Verification items for the finished model (mm, model axes). Coordinates: 2 decimals unless noted, no trailing zeros. Write each loop counter-clockwise with the first axis right and the second up, starting at its lowest first coordinate (ties: lowest second). Pieces come first, ordered by that corner, then holes. Notation, with made-up numbers: (-14.75, 57) -> (2.25, 57) arc R15 cw to (2.25, 71) -> close; hole circle Ø5 at (24.5, 5.5). An arc over 180 degrees is marked (long way). Write item = value, one per line. Start each with the question number.
(1) Section check A-A (y = 108). Record the cut outline in (x, z), plus the area to 3 significant figures.
(2) Material ranges on probe 1 along X at (y, z) = (466, 1.35); probe 2 along Y at (x, z) = (5, 3.15); probe 3 along X at (y, z) = (321, 2.1), recorded low to high. Write a range as [from, to].
(3) Gauge pin test, flat end, axial feed: pin 1 Ø2.5 at (x, y) = (160, 208) entering from -Z. Record the tip position at first contact, or that the pin passes through.
(4) Section check B-B (y = 443). Record the cut outline in (x, z).
(5) Section check C-C (z = 2.2). State how many separate pieces and enclosed holes the cut face has, plus the area to 3 significant figures.
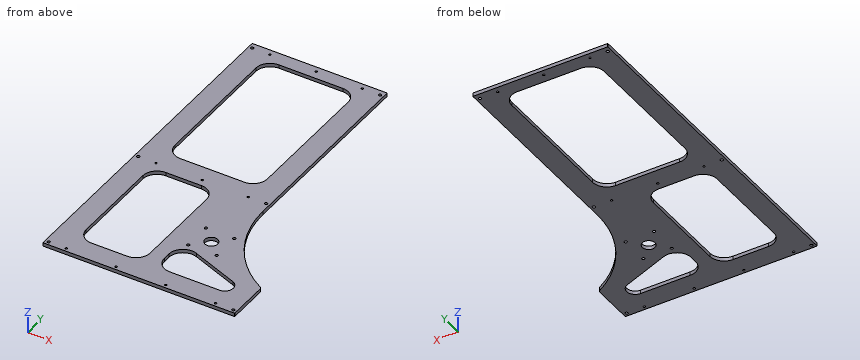
```python
from build123d import *

# Parameters (mm, degrees)
SKETCH1_R          = 9
EXTRUDE1_DEPTH     = 5
SKETCH2_R          = 2
SKETCH2_R_2        = 1.5
CUT_EXTRUDE1_DEPTH = 546.528184423
FILLET1_R          = 3
FILLET2_R          = 0.5
SKETCH3_R          = 2
CUT_EXTRUDE2_DEPTH = 546.528184423


with BuildPart() as part:
    # Sketch1 → Extrude1 (new body)
    with BuildSketch(Plane.XY):
        with BuildLine():
            Line((0, 0), (0, 474))
            Line((0, 474), (190, 474))
            Line((190, 474), (190, 193))
            ThreePointArc((190, 193), (211.541001234, 115.396842848), (270, 60))
            Line((270, 60), (270, 0))
            Line((270, 0), (0, 0))
        make_face()
        with Locations((170, 108)):
            Circle(SKETCH1_R, mode=Mode.SUBTRACT)
        with BuildLine():
            Line((30, 434), (30, 251))
            ThreePointArc((30, 251), (35.857864376, 236.857864376), (50, 231))
            Line((50, 231), (140, 231))
            ThreePointArc((140, 231), (154.142135624, 236.857864376), (160, 251))
            Line((160, 251), (160, 434))
            ThreePointArc((160, 434), (154.142135624, 448.142135624), (140, 454))
            Line((140, 454), (50, 454))
            ThreePointArc((50, 454), (35.857864376, 448.142135624), (30, 434))
        make_face(mode=Mode.SUBTRACT)
        with BuildLine():
            Line((30, 178), (30, 50))
            ThreePointArc((30, 50), (35.857864376, 35.857864376), (50, 30))
            Line((50, 30), (100, 30))
            ThreePointArc((100, 30), (114.142135624, 35.857864376), (120, 50))
            Line((120, 50), (120, 178))
            ThreePointArc((120, 178), (114.142135624, 192.142135624), (100, 198))
            Line((100, 198), (50, 198))
            ThreePointArc((50, 198), (35.857864376, 192.142135624), (30, 178))
        make_face(mode=Mode.SUBTRACT)
        with BuildLine():
            Line((160, 30), (230, 30))
            ThreePointArc((230, 30), (241.803319166, 39.836286369), (234.256500428, 53.219723887))
            Line((234.256500428, 53.219723887), (167.09416738, 78.699539812))
            ThreePointArc((167.09416738, 78.699539812), (148.639615931, 76.460306006), (140, 60))
            Line((140, 60), (140, 50))
            ThreePointArc((140, 50), (145.857864376, 35.857864376), (160, 30))
        make_face(mode=Mode.SUBTRACT)
    extrude(amount=EXTRUDE1_DEPTH)

    # Sketch2 → Cut-Extrude1 (cut, through all)
    with BuildSketch(Plane.XY.offset(5)):
        with Locations((185, 466)):
            Circle(SKETCH2_R)
        with Locations((5, 466)):
            Circle(SKETCH2_R)
        with Locations((5, 208)):
            Circle(SKETCH2_R)
        with Locations((5, 5)):
            Circle(SKETCH2_R)
        with Locations((265, 5)):
            Circle(SKETCH2_R)
        with Locations((185, 208)):
            Circle(SKETCH2_R)
        with Locations((30, 5)):
            Circle(SKETCH2_R_2)
        with Locations((100, 5)):
            Circle(SKETCH2_R_2)
        with Locations((170, 5)):
            Circle(SKETCH2_R_2)
        with Locations((240, 5)):
            Circle(SKETCH2_R_2)
        with Locations((30, 208)):
            Circle(SKETCH2_R_2)
        with Locations((95, 208)):
            Circle(SKETCH2_R_2)
        with Locations((160, 208)):
            Circle(SKETCH2_R_2)
        with Locations((30, 466)):
            Circle(SKETCH2_R_2)
        with Locations((95, 466)):
            Circle(SKETCH2_R_2)
        with Locations((160, 466)):
            Circle(SKETCH2_R_2)
    extrude(amount=-CUT_EXTRUDE1_DEPTH, mode=Mode.SUBTRACT)

    # Fillet1
    fillet1_edges = [part.edges().sort_by_distance(p)[0] for p in [
        (270, 60, 2.5),
    ]]
    fillet(fillet1_edges, radius=FILLET1_R)

    # Fillet2
    fillet2_edges = [part.edges().sort_by_distance(p)[0] for p in [
        (190, 474, 2.5),
        (270, 0, 2.5),
        (0, 0, 2.5),
        (0, 474, 2.5),
    ]]
    fillet(fillet2_edges, radius=FILLET2_R)

    # Sketch3 → Cut-Extrude2 (cut, through all)
    with BuildSketch(Plane.XY.offset(5)):
        with Locations((150, 128)):
            Circle(SKETCH3_R)
        with Locations((190, 128)):
            Circle(SKETCH3_R)
        with Locations((150, 88)):
            Circle(SKETCH3_R)
        with Locations((190, 88)):
            Circle(SKETCH3_R)
    extrude(amount=-CUT_EXTRUDE2_DEPTH, mode=Mode.SUBTRACT)


solid = part.part
```
Response:
q1.outline = (0, 0) -> (30, 0) -> (30, 5) -> (0, 5) -> close; (120, 0) -> (161, 0) -> (161, 5) -> (120, 5) -> close; (179, 0) -> (216.29, 0) -> (216.29, 5) -> (179, 5) -> close
q1.area = 541 mm2
q2.probe_1 = [0, 3], [7, 28.5], [31.5, 93.5], [96.5, 158.5], [161.5, 183], [187, 190]
q2.probe_2 = [0, 3], [7, 206], [210, 464], [468, 474]
q2.probe_3 = [0, 30], [160, 190]
q3.pin_1 = through
q4.outline = (0, 0) -> (32.14, 0) -> (32.14, 5) -> (0, 5) -> close; (157.86, 0) -> (190, 0) -> (190, 5) -> (157.86, 5) -> close
q5.separate_pieces = 1
q5.enclosed_holes = 24
q5.area = 50,300 mm2
